Autodesk Inventor part; units mm, degrees
ref_plane "Work Plane1" through (0, 0, 0) normal (1, 0, 0) x (0, 1, 0)
ref_plane "XZ Plane" through (0, 0, 0) normal (0, 1, 0) x (-1, 0, 0)
ref_plane "XY Plane" through (0, 0, 0) normal (0, 0, 1) x (1, 0, 0)
sketch "Sketch2" plane through (0, 0, 0) normal (0, 0, 1) x (1, 0, 0)
  circle A0 centre (0, 0) radius 3.15
  line L0 (-8.5, -10.15) -> (-8.5, 0)
  line L1 (8.5, 0) -> (8.5, -10.15)
  line L2 (-8.5, -10.15) -> (8.5, -10.15)
  arc A1 (8.5, 0) -> (-8.5, 0) centre (0, 0) ccw
  line L3 (0, 8.5) -> (8.5, 8.5) construction
  dimension "d0" = 6.3
  dimension "d1" = 17
  dimension "d2" = 18.65
extrude "Extrusion1" add sketch "Sketch2" along normal blind 6.5
sketch "Sketch3" plane through (-8.5, -10.15, 0) normal (0, -1, 0) x (1, 0, 0)
  line L0 (0, 6.5) -> (17, 6.5)
  line L1 (0, 0) -> (0, 6.5)
  circle A0 centre (8.5, 3.25) radius 26.7
  point P0 (8.5, 0)
  point P1 (0, 3.25)
  point P2 (0, 3.25)
  point P3 (8.5, 6.5)
  dimension "d5" = 53.4
extrude "Extrusion2" add sketch "Sketch3" along normal blind 23
sketch "Sketch4" plane through (0, 0, 0) normal (0, 0, -1) x (-1, 0, 0)
  circle A0 centre (0, 0) radius 3.15
  circle A1 centre (0, 0) radius 3.15
  arc A2 (8.5, 0) -> (-8.5, 0) centre (0, 0) ccw
  line L0 (8.5, 0) -> (8.5, -10.15)
  line L1 (8.5, -10.15) -> (26.5015, -10.15)
  line L2 (26.5015, -10.15) -> (26.5015, -33.15)
  line L3 (26.5015, -33.15) -> (-26.5015, -33.15)
  line L4 (-26.5015, -33.15) -> (-26.5015, -10.15)
  line L5 (-26.5015, -10.15) -> (-8.5, -10.15)
  line L6 (-8.5, -10.15) -> (8.5, -10.15)
  line L7 (-8.5, -10.15) -> (-8.5, 0)
  circle A3 centre (0, -18.5) radius 4.76
  dimension "d8" = 9.52
  dimension "d9" = 8.35
extrude "Extrusion3" add sketch "Sketch4" along normal blind 46 contours A3
sketch "Sketch5" plane through (0, -18.5, -46) normal (0, 0, -1) x (-1, 0, 0)
  circle A0 centre (0, 0) radius 4.76
  circle A1 centre (0, 0) radius 2.25
  point P0 (0, 18.5)
  dimension "d12" = 4.5
extrude "Extrusion4" add sketch "Sketch5" along normal blind 32 contours A1
ref_plane "Work Plane1" through (0, 0, 0) normal (1, 0, 0) x (0, 1, 0)
properties part number "dial-indicator"
Geometry: final body of the model. Coordinates: model frame, mm. A direction names the side the tool comes from. Give positions to 0.01 mm unless a question says otherwise; leave off trailing zeros. Loops run counter-clockwise (first coordinate to the right, second up) from the corner with the lowest first, then second, coordinate; pieces in that order, holes last. Notation, with made-up numbers: M -15.75,3.25 L 5.25,3.25 A20 ccw 5.25,28.25 Z; hole C 82,-0.75 d4. An arc over 180 degrees is marked long. Put each result on its own line as item: value. Start each with the question number.
1) Cut plane A-A (x = 0). Output: boundary loops of the cut face in (y, z), then the cut area to 3 significant figures.
2) Pull-direction query (X, two-part tool) for faces 5 (the cylindrical face through (-2.5, 1.917, 3.204)), 6 (the flat face through (8.5, -5, 3)), 7 (the flat face through (0, -18, -78)); classes: pulls with the +X half, pulls with the -X half, needs draft (parallel to the pull), parting line crosses it, or undercut.
3) Cut plane C-C (y = -18.5). Output: boundary loops of the cut face in (x, z), then the cut area to 3 significant figures.
4) Cut plane B-B (z = 3.25). Output: boundary loops of the cut face in (x, y), then the cut area to 3 significant figures.
5) Cut plane D-D (z = -57). Output: boundary loops of the cut face in (x, y), then the cut area to 3 significant figures.
6) Contact query for flat-ended pins moving along their axis: pin 1 (8 mm diameter, centred on y = -10, z = -7, fed in from -X); pin 2 (5 mm diameter, centred on x = -1.5, y = -3.5, fed in from +Z); pin 3 (4 mm diameter, centred on y = -20.5, z = -8.5, fed in from -X). Output: stop coordinate, or through.
7) Ray query, line 1 along Y through (x, z) = (0, 3); line 2 along Y through (x, z) = (4, -13); line 3 along X through (y, z) = (-18, -17.5). Return the intervals inside material, ascending.
8) Access query for faces 1 (the cylindrical face through (-2.2, -14.28, -34.35)), 2 (the flat face through (-8.5, -5, 3)), 3 (the flat face through (2, -3, 0)), 4 (the flat face through (2, -3, 6.5)). Directions: +Z, -Z, +X, -X, +Y, -Y. A direction counts if a zero-diameter tool reaches every point of the face in a straight line with its end or side. Return the directions, or none.
Verdict:
1. outline: M -33.15,-23.45 L -23.26,-23.45 L -23.26,-46 L -20.75,-46 L -20.75,-78 L -16.25,-78 L -16.25,-46 L -13.74,-46 L -13.74,-23.45 L -10.15,-23.45 L -10.15,0 L -3.15,0 L -3.15,6.5 L -10.15,6.5 L -10.15,29.95 L -33.15,29.95 Z; M 3.15,0 L 8.5,0 L 8.5,6.5 L 3.15,6.5 Z
1. area: 1,670 mm2
2. face 5: undercut
2. face 6: pulls with the +X half
2. face 7: needs draft
3. outline: M -4.76,-46 L -2.25,-46 L -2.25,-78 L 2.25,-78 L 2.25,-46 L 4.76,-46 L 4.76,-23.02 A26.7 ccw long -4.76,-23.02 Z
3. area: 2,600 mm2
4. outline: M -26.7,-33.15 L 26.7,-33.15 L 26.7,-10.15 L 8.5,-10.15 L 8.5,0 A8.5 ccw -8.5,0 L -8.5,-10.15 L -26.7,-10.15 Z; hole C 0,0 d6.3
4. area: 1,480 mm2
5. outline: C 0,-18.5 d4.5
5. area: 15.9 mm2
6. pin 1: x = -25.96
6. pin 2: z = 6.5
6. pin 3: x = -24.86
7. line 1: -33.15 to -3.15, 3.15 to 8.5
7. line 2: -33.15 to -10.15
7. line 3: -16.8 to 16.8
8. face 1: -Z
8. face 2: +Z, -Z, -X, +Y
8. face 3: -Z, +X, -X, +Y
8. face 4: +Z, +X, -X, +Y
